For this review, take the finished solid that the model builds, in its own axes (mm). Face numbers are marked on the shaded views. A direction names the side the tool comes from. Give positions to 0.01 mm unless a question says otherwise; leave off trailing zeros. Write each loop counter-clockwise with the first axis right and the second up, starting at its lowest first coordinate (ties: lowest second). Pieces come first, ordered by that corner, then holes. Notation, with made-up numbers: M 7.25,-30.5 L 29.25,-30.5 A11 ccw 29.25,-18.5 Z; hole C 32.25,52 d3. An arc over 180 degrees is marked long. Use one line per item in the form item = value. Start each with the question number.
Q1. Consider section C-C on x = -3.5. Write out the cut boundary in (y, z).
Q2. Consider section A-A on z = 6. Write out the cut boundary in (x, y).
Q3. Tool access review of the marked faces 1, 2, 3 and 4: name each direction out of +Z, -Z, +X, -X, +Y, -Y from which nothing blocks a thin tool from reaching the whole face with its end or side.
Q4. Mouldability with a two-part tool opening along Z and no side actions: class the marked faces 5, 6, 7 and 8 as released by +Z, released by -Z, zero draft, split by the parting line, or undercut.
Q5. Consider section B-B on y = -20.5. Write out the cut boundary in (x, z).
Q6. Consider section D-D on y = 235.5. Write out the cut boundary in (x, z).
Q7. Clearance check with flat-ended pins moving along their axes: pin 1 Ø1 at (y, z) = (52, 43.5) entering from -X; pin 2 Ø10 at (x, y) = (23, 211) entering from +Z; pin 3 Ø12 at (x, z) = (-14, 83) entering from -Y. State where each tip first meets the part, or that it passes through.
Q8. For probe 1 along X at (y, z) = (-17, 38); probe 2 along X at (y, z) = (230, 49.5) (3 decimals); probe 3 along Y at (x, z) = (45, 50), list the stretches that pass through material, from the lowest coordinate up. Write a range as [from, to].
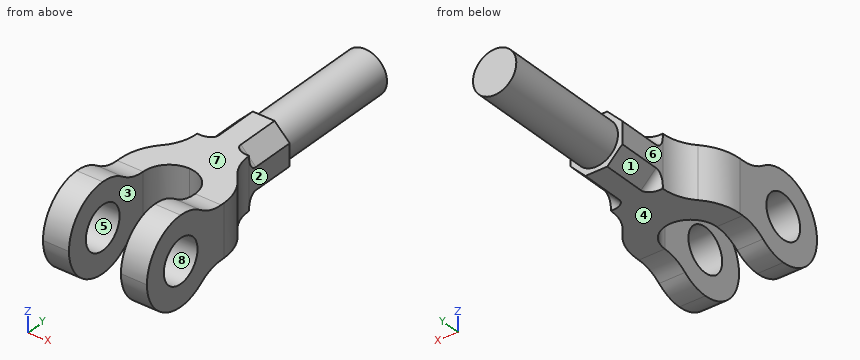
```python
from build123d import *

# Parameters (mm, degrees)
SKETCH1_W           = 120
SKETCH1_H           = 250
BOSS_EXTRUDE1_DEPTH = 100
CUT_EXTRUDE1_DEPTH  = 100
CUT_EXTRUDE2_DEPTH  = 240
SKETCH4_4_R         = 25
CUT_EXTRUDE3_DEPTH  = 240
CUT_EXTRUDE4_DEPTH  = 60
SKETCH5_3_R         = 25
BOSS_EXTRUDE2_DEPTH = 150.7
FILLET1_R           = 10


with BuildPart() as part:
    # Sketch1 → Boss-Extrude1 (new body)
    with BuildSketch(Plane.XY):
        Rectangle(SKETCH1_W, SKETCH1_H)
    extrude(amount=BOSS_EXTRUDE1_DEPTH)

    # Sketch2 → Cut-Extrude1 (cut)
    with BuildSketch(Plane.XY.offset(100)):
        with BuildLine():
            ThreePointArc((30, -15), (21.213203436, 6.213203436), (0, 15))
            ThreePointArc((0, 15), (-21.213203436, 6.213203436), (-30, -15))
            Line((-30, -15), (-30, -125))
            Line((-30, -125), (30, -125))
            Line((30, -125), (30, -15))
        make_face()
        with BuildLine():
            Line((60, 125), (30, 125))
            Line((30, 125), (30, 64.498344353))
            ThreePointArc((30, 64.498344353), (33.533981136, 46.034620706), (43.636363636, 30.180915101))
            ThreePointArc((43.636363636, 30.180915101), (55.759222645, 11.156468358), (60, -11.00000004))
            Line((60, -11.00000004), (60, 125))
        make_face()
        with BuildLine():
            Line((-30, 64.498344353), (-30, 125))
            Line((-30, 125), (-60, 125))
            Line((-60, 125), (-60, -11))
            ThreePointArc((-60, -11), (-55.759222637, 11.156468376), (-43.636363636, 30.180915101))
            ThreePointArc((-43.636363636, 30.180915101), (-33.533981136, 46.034620706), (-30, 64.498344353))
        make_face()
    extrude(amount=-CUT_EXTRUDE1_DEPTH, mode=Mode.SUBTRACT)

    # Sketch4 → Cut-Extrude2 (cut)
    with BuildSketch(Plane(origin=(70, 0, 0), x_dir=(0, 0, -1), z_dir=(1, 0, 0))):
        with BuildLine():
            Line((-100, 125), (-100, -75))
            ThreePointArc((-100, -75), (-97.434164903, -59.188611699), (-90, -45))
            ThreePointArc((-90, -45), (-82.565835097, -30.811388301), (-80, -15))
            Line((-80, -15), (-80, 125))
            Line((-80, 125), (-100, 125))
        make_face()
        with BuildLine():
            ThreePointArc((-10, -45), (-2.565835058, -59.188611819), (0, -75.000000253))
            Line((0, -75.000000253), (0, 125))
            Line((0, 125), (-20, 125))
            Line((-20, 125), (-20, -15))
            ThreePointArc((-20, -15), (-17.434164903, -30.811388301), (-10, -45))
        make_face()
        with BuildLine():
            Line((-100, -75), (-100, -125))
            Line((-100, -125), (-50, -125))
            ThreePointArc((-50, -125), (-85.355339059, -110.355339059), (-100, -75))
        make_face()
        with BuildLine():
            ThreePointArc((0, -75.000000253), (-14.64466103, -110.355339149), (-50, -125))
            Line((-50, -125), (0, -125))
            Line((0, -125), (0, -75.000000253))
        make_face()
    extrude(amount=-CUT_EXTRUDE2_DEPTH, mode=Mode.SUBTRACT)

    # Sketch4_4 → Cut-Extrude3 (cut)
    with BuildSketch(Plane(origin=(70, 0, 0), x_dir=(0, 0, -1), z_dir=(1, 0, 0))):
        with Locations((-50, -75)):
            Circle(SKETCH4_4_R)
    extrude(amount=-CUT_EXTRUDE3_DEPTH, mode=Mode.SUBTRACT)

    # Sketch5 → Cut-Extrude4 (cut)
    with BuildSketch(Plane(origin=(0, 125, 0), x_dir=(1, 0, 0), z_dir=(0, 1, 0))):
        Polygon((-30, -20), (-30, -37.4), (-12.6, -20), align=None)
        Polygon((-21.3, -71.3), (-30, -80), (-12.6, -80), align=None)
        Polygon((-30, -62.6), (-30, -80), (-21.3, -71.3), align=None)
        Polygon((30, -62.6), (12.6, -80), (30, -80), align=None)
        Polygon((12.6, -20), (21.3, -28.7), (30, -20), align=None)
        Polygon((30, -20), (21.3, -28.7), (30, -37.4), align=None)
    extrude(amount=-CUT_EXTRUDE4_DEPTH, mode=Mode.SUBTRACT)

    # Sketch5_3 → Boss-Extrude2 (add)
    with BuildSketch(Plane(origin=(0, 125, 0), x_dir=(1, 0, 0), z_dir=(0, 1, 0))):
        with Locations(Location((0, -50, 0), (0, 0, 270))):
            Circle(SKETCH5_3_R)
    extrude(amount=BOSS_EXTRUDE2_DEPTH)

    # Fillet1
    fillet1_edges = [part.edges().sort_by_distance(p)[0] for p in [
        (21.3, 65, 28.7),
        (21.3, 65, 71.3),
        (-21.3, 65, 71.3),
        (-21.3, 65, 28.7),
    ]]
    fillet(fillet1_edges, radius=FILLET1_R)


solid = part.part
```
Working result:
q1.outline = M 14.8,20 L 125,20 L 125,25.25 L 275.7,25.25 L 275.7,74.75 L 125,74.75 L 125,80 L 14.8,80 Z
q2.outline = M -60,-98.75 L -30,-98.75 L -30,-51.25 L -60,-51.25 Z; M 30,-98.75 L 60,-98.75 L 60,-51.25 L 30,-51.25 Z
q3.face_1 = -Z, -X, +Y
q3.face_2 = +Z, -Z, +X, +Y
q3.face_3 = +Z, -Z, -Y
q3.face_4 = -Z, +X, -X, +Y
q4.face_5 = undercut
q4.face_6 = zero draft
q4.face_7 = released by +Z
q4.face_8 = undercut
q5.outline = M -60,19.7 L -30,19.7 L -30,80.3 L -60,80.3 Z; M 30,19.7 L 60,19.7 L 60,80.3 L 30,80.3 Z
q6.outline = C 0,50 d50
q7.pin_1 = -31.72
q7.pin_2 = 67.35
q7.pin_3 = 8.05
q8.probe_1 = [-60, -30], [30, 60]
q8.probe_2 = [-24.995, 24.995]
q8.probe_3 = [-125, -100], [-50, 28.69]
